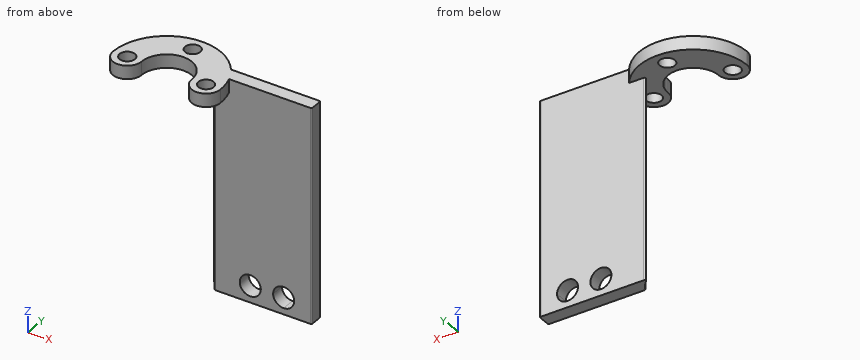
```python
from build123d import *

# Parameters (mm, degrees)
SKETCH1_R           = 1.45
BOSS_EXTRUDE1_DEPTH = 2.54
BOSS_EXTRUDE2_DEPTH = 38.1
FILLET1_R           = 0.254
CUT_EXTRUDE1_DEPTH  = 19.05


with BuildPart() as part:
    # Sketch1 → Boss-Extrude1 (new body)
    with BuildSketch(Plane.XY):
        with BuildLine():
            ThreePointArc((10.22, 0), (10.07983069, 1.686835278), (9.663167661, 3.3274))
            Line((9.663167661, 3.3274), (25.4, 3.3274))
            Line((25.4, 3.3274), (25.4, 5.8674))
            Line((25.4, 5.8674), (8.367915944, 5.8674))
            ThreePointArc((8.367915944, 5.8674), (-3.076385784, 9.745986379), (-10.22, 1.2e-08))
            ThreePointArc((-10.22, 1.2e-08), (-7.500000006, -2.72), (-4.78, 0))
            ThreePointArc((-4.78, 0), (0, 4.78), (4.78, 0))
            ThreePointArc((4.78, 0), (7.5, -2.72), (10.22, 0))
        make_face()
        with Locations((7.5, 0)):
            Circle(SKETCH1_R, mode=Mode.SUBTRACT)
        with Locations((-7.5, 0)):
            Circle(SKETCH1_R, mode=Mode.SUBTRACT)
        with Locations((0, 7.5)):
            Circle(SKETCH1_R, mode=Mode.SUBTRACT)
    extrude(amount=BOSS_EXTRUDE1_DEPTH)

    # Sketch1<3> → Boss-Extrude2 (add)
    with BuildSketch(Plane.XY):
        with BuildLine():
            ThreePointArc((4.955402833, 5.8674), (6.072863387, 4.70135409), (6.921763449, 3.3274))
            Line((6.921763449, 3.3274), (25.4, 3.3274))
            Line((25.4, 3.3274), (25.4, 5.8674))
            Line((25.4, 5.8674), (4.955402833, 5.8674))
        make_face()
    extrude(amount=-BOSS_EXTRUDE2_DEPTH)

    # Fillet1
    fillet1_edges = [part.edges().sort_by_distance(p)[0] for p in [
        (25.4, 5.8674, -17.78),
        (25.4, 3.3274, -17.78),
        (4.955402833, 5.8674, -19.05),
        (6.921763449, 3.3274, -19.05),
    ]]
    fillet(fillet1_edges, radius=FILLET1_R)

    # Sketch5 → Cut-Extrude1 (cut)
    with BuildSketch(Plane(origin=(0, 5.8674, 0), x_dir=(1, 0, 0), z_dir=(0, 1, 0))):
        with BuildLine():
            Line((22.06625, 34.925), (20.066, 34.925))
            Line((20.066, 34.925), (18.06575, 34.925))
            ThreePointArc((18.06575, 34.925), (20.066, 32.92475), (22.06625, 34.925))
        make_face()
        with BuildLine():
            ThreePointArc((22.06625, 34.925), (21.480390339, 36.339390339), (20.066, 36.92525))
            Line((20.066, 36.92525), (20.066, 34.925))
            Line((20.066, 34.925), (22.06625, 34.925))
        make_face()
        with BuildLine():
            Line((20.066, 34.925), (20.066, 36.92525))
            ThreePointArc((20.066, 36.92525), (18.651609661, 36.339390339), (18.06575, 34.925))
            Line((18.06575, 34.925), (20.066, 34.925))
        make_face()
        with BuildLine():
            ThreePointArc((15.71625, 34.925), (13.716, 36.92525), (11.71575, 34.925))
            Line((11.71575, 34.925), (15.71625, 34.925))
        make_face()
        with BuildLine():
            Line((15.71625, 34.925), (11.71575, 34.925))
            ThreePointArc((11.71575, 34.925), (13.716, 32.92475), (15.71625, 34.925))
        make_face()
    extrude(amount=-CUT_EXTRUDE1_DEPTH, mode=Mode.SUBTRACT)


solid = part.part
```
For this review, take the finished solid that the model builds, in its own axes (mm). Round coordinates to 2 decimals unless told otherwise and drop trailing zeros. Loops run counter-clockwise (first coordinate to the right, second up) from the corner with the lowest first, then second, coordinate; pieces in that order, holes last.
(1) We need section B-B (y = 2.25). Give the boundary of the cut face in (x, z).
Returned:
outline: (-9.97, 0) - (-4.22, 0) - (-4.22, 2.54) - (-9.97, 2.54) - close; (4.22, 0) - (9.97, 0) - (9.97, 2.54) - (4.22, 2.54) - close
(2) Wall thickness on line 1 along Z through (x, y) = (13.5, 3.5); line 2 along Y through (x, z) = (0, 1); line 3 along Z through (x, y) = (6, 0.25): over which ranges is each line inside the solid? List them lowest first.
Returned:
line 1: z = -38.1 to -36.91, -32.94 to 2.54
line 2: y = 4.78 to 6.05, 8.95 to 10.22
line 3: z = 0 to 2.54
(3) Clearance check with flat-ended pins moving along their axes: P1, Ø20, axis at x = 13.5, z = -25, coming from the -Y side; P2, Ø3.5, axis at x = 7.5, y = 0, coming from the +Z side; P3, Ø12, axis at x = 12, z = -34, coming from the +Y side; P4, Ø6, axis at x = 14.5, y = -0.5, coming from the +Z side. State where each tip first meets the part, or that it passes through.
Returned:
P1: stops at y = 3.33
P2: stops at z = 2.54
P3: stops at y = 5.87
P4: passes through
(4) We need section D-D (z = -10). Give the boundary of the cut face in (x, y).
Returned:
outline: (5.43, 5.43) arc R7.68 cw to (6.85, 3.47) arc R0.25 ccw to (7.08, 3.33) - (25.15, 3.33) arc R0.25 ccw to (25.4, 3.58) - (25.4, 5.61) arc R0.25 ccw to (25.15, 5.87) - (5.61, 5.87) arc R0.25 ccw to start
(5) We need section A-A (x = 0). Give the boundary of the cut face in (y, z).
Returned:
outline: (4.78, 0) - (6.05, 0) - (6.05, 2.54) - (4.78, 2.54) - close; (8.95, 0) - (10.22, 0) - (10.22, 2.54) - (8.95, 2.54) - close
(6) We need section C-C (y = -0.5). Give the boundary of the cut face in (x, z), plus the area to 3 significant figures.
Returned:
outline: (-10.17, 0) - (-8.86, 0) - (-8.86, 2.54) - (-10.17, 2.54) - close; (-6.14, 0) - (-4.83, 0) - (-4.83, 2.54) - (-6.14, 2.54) - close; (4.83, 0) - (6.14, 0) - (6.14, 2.54) - (4.83, 2.54) - close; (8.86, 0) - (10.17, 0) - (10.17, 2.54) - (8.86, 2.54) - close
area: 13.3 mm2
